Model file for the job. Use its own axes, mm. Coordinates: 2 decimals unless noted, no trailing zeros. Loops run counter-clockwise (first coordinate to the right, second up) from the corner with the lowest first, then second, coordinate; pieces in that order, holes last.
Autodesk Inventor part; units mm, degrees
ref_plane "YZ Plane" through (0, 0, 0) normal (1, 0, 0) x (0, 1, 0)
ref_plane "XZ Plane" through (0, 0, 0) normal (0, 1, 0) x (-1, 0, 0)
ref_plane "XY Plane" through (0, 0, 0) normal (0, 0, 1) x (1, 0, 0)
sketch "Sketch1" plane through (0, 0, 0) normal (0, 1, 0) x (-1, 0, 0)
  line L0 (-9.525, -9.525) -> (9.525, -9.525)
  line L1 (9.525, -9.525) -> (9.525, 9.525)
  line L2 (9.525, 9.525) -> (-9.525, 9.525)
  line L3 (-9.525, 9.525) -> (-9.525, -9.525)
  line L4 (-9.525, -9.525) -> (9.525, 9.525) construction
  line L5 (9.525, -9.525) -> (-9.525, 9.525) construction
  point P0 (0, 0)
  dimension "d0" = 19.05
  dimension "d1" = 19.05
sketch "Sketch2" plane through (0, 0, 0) normal (1, 0, 0) x (0, 1, 0)
  line L0 (0, 0) -> (112.776, 25.4)
  dimension "d2" = 112.776
  dimension "d3" = 25.4
sweep "Sweep1" add profiles "Sketch1" path "Sketch2"
sketch "Sketch3" plane through (-9.525, 112.776, 34.925) normal (0, 1, 0) x (1, 0, 0)
  line L0 (34.925, 76.2) -> (-15.875, 76.2)
  line L1 (-15.875, 76.2) -> (-15.875, -25.4)
  line L2 (-15.875, -25.4) -> (34.925, -25.4)
  line L3 (34.925, -25.4) -> (34.925, 76.2)
  line L4 (0, 25.4) -> (19.05, 25.4)
  line L5 (34.925, 76.2) -> (-15.875, -25.4) construction
  line L6 (-15.875, 76.2) -> (34.925, -25.4) construction
  point P0 (9.525, 34.925)
  point P1 (9.525, 25.4)
  dimension "d6" = 50.8
  dimension "d7" = 101.6
extrude "Extrusion1" cut sketch "Sketch3" against normal blind 49.276
sketch "Sketch4" plane through (-9.525, 0, -9.525) normal (0, -1, 0) x (1, 0, 0)
  circle A0 centre (9.525, 9.525) radius 2.413
  dimension "d10" = 4.826
extrude "Extrusion2" cut sketch "Sketch4" against normal blind 19.05
thread "Thread1"
sketch "Sketch5" plane through (-9.525, 63.5, 34.925) normal (0, 1, 0) x (1, 0, 0)
  circle A0 centre (9.525, 20.6232) radius 2.413
  line L0 (0, 11.0982) -> (0, 30.1482)
  line L1 (19.05, 11.0982) -> (0, 11.0982)
  point P0 (9.525, 34.925)
  point P1 (0, 20.6232)
  point P2 (9.525, 11.0982)
  dimension "d15" = 4.826
extrude "Extrusion3" cut sketch "Sketch5" against normal blind 19.05
properties part number "STRU_008_BilletBlock_Slanted"
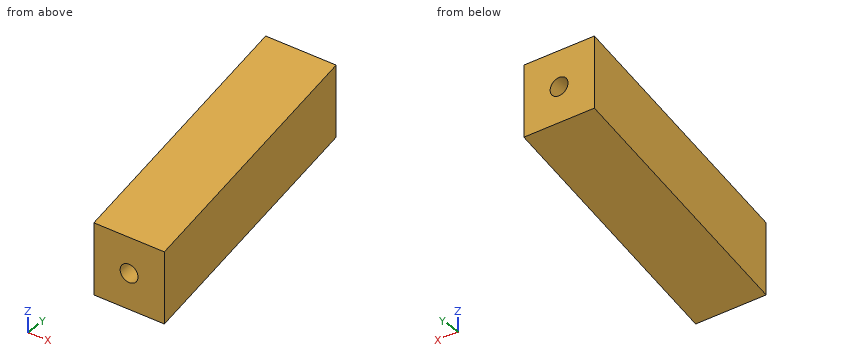
Q1. Drill centre lines: line 1 (X direction, y = 44.5, z = 14.5) (3 decimals); line 2 (Z direction, x = 0, y = 14); line 3 (Z direction, x = 8.75, y = 14). Where is each one in solid material? Low to high.
Answers:
line 1: x = -9.525 to -2.405, 2.405 to 9.525
line 2: z = -6.37 to -2.41, 2.41 to 12.68
line 3: z = -6.37 to 12.68
Q2. Slice it at B-B (z = -1). List the corners of the cut face in (x, y) (3 decimals), and give its area (3 significant figures).
Answers:
outline: (-9.525, 0) - (-2.196, 0) - (-2.196, 19.05) - (2.196, 19.05) - (2.196, 0) - (9.525, 0) - (9.525, 37.851) - (-9.525, 37.851) - close
area: 637 mm2
Q3. Slice it at C-C (y = 46). List the corners of the cut face in (x, z) (3 decimals).
Answers:
outline: (-9.525, 0.835) - (9.525, 0.835) - (9.525, 19.885) - (-9.525, 19.885) - close; hole circle Ø4.826 at (0, 14.302)
Q4. Slice it at D-D (x = -4.75). List the corners of the cut face in (y, z) (3 decimals), and give its area (3 significant figures).
Answers:
outline: (0, -9.525) - (63.5, 4.777) - (63.5, 23.827) - (0, 9.525) - close
area: 1,210 mm2
Q5. Slice it at A-A (x = 0). List the corners of the cut face in (y, z) (3 decimals), and give its area (3 significant figures).
Answers:
outline: (0, -9.525) - (63.5, 4.777) - (63.5, 11.889) - (44.45, 11.889) - (44.45, 16.715) - (63.5, 16.715) - (63.5, 23.827) - (0, 9.525) - (0, 2.413) - (19.05, 2.413) - (19.05, -2.413) - (0, -2.413) - close
area: 1,030 mm2
Q6. Flat gauge pins, fed straight in: P1, Ø5, axis at x = -4, y = 15, coming from the -Z side; P2, Ø1.4, axis at x = 0.5, z = 0, coming from the -Y side; P3, Ø5, axis at x = -6.5, y = 18, coming from the -Z side. Where does each tip first touch, or does it go through?
Answers:
P1: stops at z = -6.71
P2: stops at y = 19.05
P3: stops at z = -6.03
